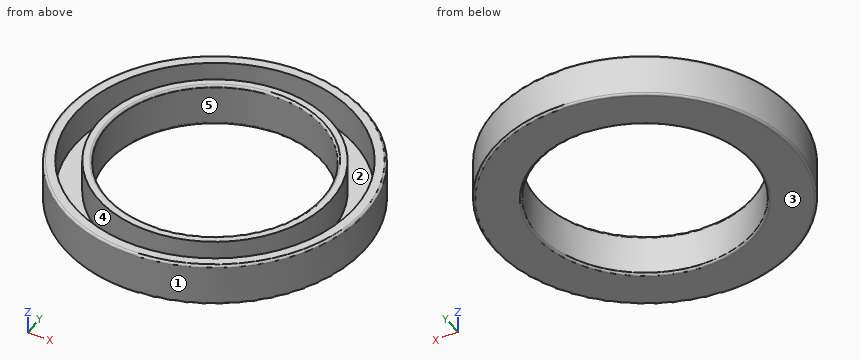
```python
from build123d import *

# Parameters (mm, degrees)
SKETCH1_R           = 35
SKETCH1_R_2         = 25
BOSS_EXTRUDE1_DEPTH = 10
SKETCH2_R           = 32.5
SKETCH2_R_2         = 27
CUT_EXTRUDE1_DEPTH  = 8
FILLET1_R           = 0.5


with BuildPart() as part:
    # Sketch1 → Boss-Extrude1 (new body)
    with BuildSketch(Plane.XY):
        Circle(SKETCH1_R)
        Circle(SKETCH1_R_2, mode=Mode.SUBTRACT)
    extrude(amount=BOSS_EXTRUDE1_DEPTH)

    # Sketch2 → Cut-Extrude1 (cut)
    with BuildSketch(Plane.XY.offset(10)):
        Circle(SKETCH2_R)
        Circle(SKETCH2_R_2, mode=Mode.SUBTRACT)
    extrude(amount=-CUT_EXTRUDE1_DEPTH, mode=Mode.SUBTRACT)

    # Fillet1
    fillet1_edges = [part.edges().sort_by_distance(p)[0] for p in [
        (-35, 0, 0),
        (-35, 0, 10),
        (-25, 0, 0),
        (-25, 0, 10),
    ]]
    fillet(fillet1_edges, radius=FILLET1_R)


solid = part.part
```
Input: part model. Units: mm. Frame: model coordinates. Face numbers are marked on the shaded views. A direction names the side the tool comes from. Coordinates: 2 decimals unless noted, no trailing zeros. Order: outer loops, then holes, each group sorted by start corner. A loop starts at its lowest first (then second) coordinate and runs counter-clockwise, first axis right, second up. Notation, with made-up numbers: (30.25, -4) - (66.25, -4) arc R10 cw to (66.25, 6) - close; hole circle Ø8 at (50, 82.5). An arc over 180 degrees is marked (long way). Put each result on its own line as item: value.
1. Reachability of the marked faces 4 and 5 from +Z, -Z, +X, -X, +Y, -Y: full face, straight path, thin tool, end or side. Return the list, or none.
Report:
face 4: +Z
face 5: +Z, -Z
2. Contact query for flat-ended pins moving along their axis: pin 1 Ø6 at (x, z) = (-7.5, 1.5) entering from -Y; pin 2 Ø3 at (y, z) = (27, 1) entering from +X; pin 3 Ø4 at (y, z) = (-25.5, 3) entering from +X. Output: stop coordinate, or through.
Report:
pin 1: stops at y = -34.71
pin 2: stops at x = 23.97
pin 3: stops at x = 25.94
3. Cut plane A-A on y = 0. Return the cut outline in (x, z).
Report:
outline: (-35, 0.5) arc R0.5 ccw to (-34.5, 0) - (-25.5, 0) arc R0.5 ccw to (-25, 0.5) - (-25, 9.5) arc R0.5 ccw to (-25.5, 10) - (-27, 10) - (-27, 2) - (-32.5, 2) - (-32.5, 10) - (-34.5, 10) arc R0.5 ccw to (-35, 9.5) - close; (25, 0.5) arc R0.5 ccw to (25.5, 0) - (34.5, 0) arc R0.5 ccw to (35, 0.5) - (35, 9.5) arc R0.5 ccw to (34.5, 10) - (32.5, 10) - (32.5, 2) - (27, 2) - (27, 10) - (25.5, 10) arc R0.5 ccw to (25, 9.5) - close
4. Draft query along X for the marked faces 1, 2 and 3. Return one class per face: pulls with the +X half, pulls with the -X half, needs draft (parallel to the pull), parting line crosses it, or undercut.
Report:
face 1: parting line crosses it
face 2: undercut
face 3: needs draft
5. Cut plane C-C on z = 8. Return the cut outline in (x, y), then the cut area to 3 significant figures.
Report:
outline: circle Ø70 at (0, 0); circle Ø54 at (0, 0); hole circle Ø65 at (0, 0); hole circle Ø50 at (0, 0)
area: 857 mm2
6. Line query: line 1 along Y through (x, z) = (0, 7.25); line 2 along Y through (x, z) = (-13, 9.5); line 3 along X through (y, z) = (-7.5, 7.25). Output: solid intervals per line, ascending.
Report:
line 1: y = -35 to -32.5, -27 to -25, 25 to 27, 32.5 to 35
line 2: y = -32.5 to -29.79, -23.66 to -21.35, 21.35 to 23.66, 29.79 to 32.5
line 3: x = -34.19 to -31.62, -25.94 to -23.85, 23.85 to 25.94, 31.62 to 34.19
